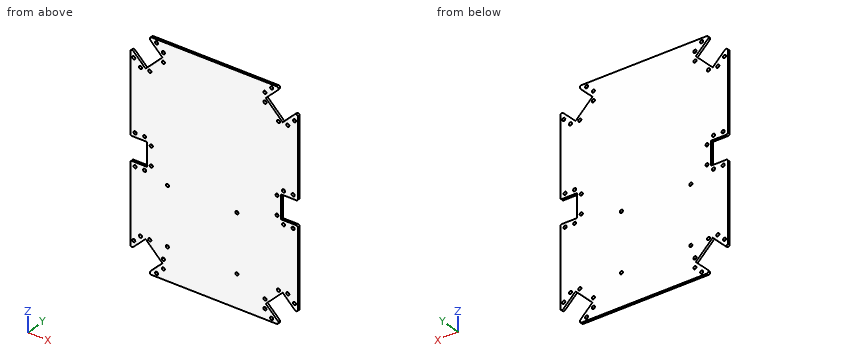
```python
from build123d import *

# Parameters (mm, degrees)
SKETCH2_W           = 140
SKETCH2_H           = 190
SKETCH2_R           = 1.3
BOSS_EXTRUDE1_DEPTH = 2
SKETCH3_W           = 14
SKETCH3_H           = 20
CUT_EXTRUDE1_DEPTH  = 2
FILLET1_R           = 1.5
SKETCH4_R           = 1.3
CUT_EXTRUDE2_DEPTH  = 2


with BuildPart() as part:
    # Sketch2 → Boss-Extrude1 (new body)
    with BuildSketch(Plane(origin=(0, 0, 0), x_dir=(1, 0, 0), z_dir=(0, 1, 0))):
        Rectangle(SKETCH2_W, SKETCH2_H)
        with Locations(Location((42.422835534, 78.736544033, 0), (0, 0, 270))):
            Circle(SKETCH2_R, mode=Mode.SUBTRACT)
        with Locations(Location((42.422835534, 86.514718626, 0), (0, 0, 270))):
            Circle(SKETCH2_R, mode=Mode.SUBTRACT)
        with Locations(Location((48.079689783, 92.171572875, 0), (0, 0, 270))):
            Circle(SKETCH2_R, mode=Mode.SUBTRACT)
        with Locations(Location((66, 13.5, 0), (0, 0, 270))):
            Circle(SKETCH2_R, mode=Mode.SUBTRACT)
        with Locations(Location((58, 13.5, 0), (0, 0, 270))):
            Circle(SKETCH2_R, mode=Mode.SUBTRACT)
        with Locations(Location((52.5, 8, 0), (0, 0, 270))):
            Circle(SKETCH2_R, mode=Mode.SUBTRACT)
        with Locations(Location((52.5, -8, 0), (0, 0, 90))):
            Circle(SKETCH2_R, mode=Mode.SUBTRACT)
        with Locations(Location((58, -13.5, 0), (0, 0, 90))):
            Circle(SKETCH2_R, mode=Mode.SUBTRACT)
        with Locations(Location((66, -13.5, 0), (0, 0, 90))):
            Circle(SKETCH2_R, mode=Mode.SUBTRACT)
        with Locations(Location((67.171572875, 73.079689783, 0), (0, 0, 90))):
            Circle(SKETCH2_R, mode=Mode.SUBTRACT)
        with Locations(Location((61.514718626, 67.422835534, 0), (0, 0, 90))):
            Circle(SKETCH2_R, mode=Mode.SUBTRACT)
        with Locations(Location((53.736544033, 67.422835534, 0), (0, 0, 90))):
            Circle(SKETCH2_R, mode=Mode.SUBTRACT)
        with Locations(Location((67.171572875, -73.079689783, 0), (0, 0, 270))):
            Circle(SKETCH2_R, mode=Mode.SUBTRACT)
        with Locations(Location((61.514718626, -67.422835534, 0), (0, 0, 270))):
            Circle(SKETCH2_R, mode=Mode.SUBTRACT)
        with Locations(Location((53.736544033, -67.422835534, 0), (0, 0, 270))):
            Circle(SKETCH2_R, mode=Mode.SUBTRACT)
        with Locations(Location((48.079689783, -92.171572875, 0), (0, 0, 90))):
            Circle(SKETCH2_R, mode=Mode.SUBTRACT)
        with Locations(Location((42.422835534, -86.514718626, 0), (0, 0, 90))):
            Circle(SKETCH2_R, mode=Mode.SUBTRACT)
        with Locations(Location((42.422835534, -78.736544033, 0), (0, 0, 90))):
            Circle(SKETCH2_R, mode=Mode.SUBTRACT)
        with Locations(Location((-48.079689783, 92.171572875, 0), (0, 0, 90))):
            Circle(SKETCH2_R, mode=Mode.SUBTRACT)
        with Locations(Location((-42.422835534, 86.514718626, 0), (0, 0, 90))):
            Circle(SKETCH2_R, mode=Mode.SUBTRACT)
        with Locations(Location((-42.422835534, 78.736544033, 0), (0, 0, 90))):
            Circle(SKETCH2_R, mode=Mode.SUBTRACT)
        with Locations(Location((-67.171572875, 73.079689783, 0), (0, 0, 270))):
            Circle(SKETCH2_R, mode=Mode.SUBTRACT)
        with Locations(Location((-61.514718626, 67.422835534, 0), (0, 0, 270))):
            Circle(SKETCH2_R, mode=Mode.SUBTRACT)
        with Locations(Location((-53.736544033, 67.422835534, 0), (0, 0, 270))):
            Circle(SKETCH2_R, mode=Mode.SUBTRACT)
        with Locations(Location((-67.171572875, -73.079689783, 0), (0, 0, 90))):
            Circle(SKETCH2_R, mode=Mode.SUBTRACT)
        with Locations(Location((-61.514718626, -67.422835534, 0), (0, 0, 90))):
            Circle(SKETCH2_R, mode=Mode.SUBTRACT)
        with Locations(Location((-53.736544033, -67.422835534, 0), (0, 0, 90))):
            Circle(SKETCH2_R, mode=Mode.SUBTRACT)
        with Locations(Location((-42.422835534, -78.736544033, 0), (0, 0, 270))):
            Circle(SKETCH2_R, mode=Mode.SUBTRACT)
        with Locations(Location((-42.422835534, -86.514718626, 0), (0, 0, 270))):
            Circle(SKETCH2_R, mode=Mode.SUBTRACT)
        with Locations(Location((-48.079689783, -92.171572875, 0), (0, 0, 270))):
            Circle(SKETCH2_R, mode=Mode.SUBTRACT)
        with Locations(Location((-52.5, -8, 0), (0, 0, 270))):
            Circle(SKETCH2_R, mode=Mode.SUBTRACT)
        with Locations(Location((-58, -13.5, 0), (0, 0, 270))):
            Circle(SKETCH2_R, mode=Mode.SUBTRACT)
        with Locations(Location((-66, -13.5, 0), (0, 0, 270))):
            Circle(SKETCH2_R, mode=Mode.SUBTRACT)
        with Locations(Location((-66, 13.5, 0), (0, 0, 90))):
            Circle(SKETCH2_R, mode=Mode.SUBTRACT)
        with Locations(Location((-58, 13.5, 0), (0, 0, 90))):
            Circle(SKETCH2_R, mode=Mode.SUBTRACT)
        with Locations(Location((-52.5, 8, 0), (0, 0, 90))):
            Circle(SKETCH2_R, mode=Mode.SUBTRACT)
    extrude(amount=BOSS_EXTRUDE1_DEPTH)

    # Sketch3 → Cut-Extrude1 (cut)
    with BuildSketch(Plane(origin=(0, 2, 0), x_dir=(1, 0, 0), z_dir=(0, 1, 0))):
        with Locations((63, 0)):
            Rectangle(SKETCH3_W, SKETCH3_H)
        Polygon((55.857864376, 95), (43.129942315, 82.272077939), (57.272077939, 68.129942315), (70, 80.857864376), (70, 95), align=None)
        Polygon((70, -80.857864376), (70, -95), (55.857864376, -95), (43.129942315, -82.272077939), (57.272077939, -68.129942315), align=None)
        Polygon((-70, 80.857864376), (-70, 95), (-55.857864376, 95), (-43.129942315, 82.272077939), (-57.272077939, 68.129942315), align=None)
        with Locations((-63, 0)):
            Rectangle(SKETCH3_W, SKETCH3_H)
        Polygon((-57.272077939, -68.129942315), (-70, -80.857864376), (-70, -95), (-55.857864376, -95), (-43.129942315, -82.272077939), align=None)
    extrude(amount=-CUT_EXTRUDE1_DEPTH, mode=Mode.SUBTRACT)

    # Fillet1
    fillet1_edges = [part.edges().sort_by_distance(p)[0] for p in [
        (55.857864376, 1, -95),
        (70, 1, -80.857864376),
        (70, 1, 80.857864376),
        (55.857864376, 1, 95),
        (-70, 1, -80.857864376),
        (-55.857864376, 1, -95),
        (-70, 1, 10),
        (-70, 1, -10),
        (-55.857864376, 1, 95),
        (-70, 1, 80.857864376),
        (70, 1, -10),
        (70, 1, 10),
    ]]
    fillet(fillet1_edges, radius=FILLET1_R)

    # Sketch4 → Cut-Extrude2 (cut)
    with BuildSketch(Plane(origin=(0, 2, 0), x_dir=(1, 0, 0), z_dir=(0, 1, 0))):
        with Locations(Location((-39, 67.5, 0), (0, 0, 270))):
            Circle(SKETCH4_R)
        with Locations(Location((19, 67.5, 0), (0, 0, 270))):
            Circle(SKETCH4_R)
        with Locations(Location((19, 18.5, 0), (0, 0, 270))):
            Circle(SKETCH4_R)
        with Locations(Location((-39, 18.5, 0), (0, 0, 270))):
            Circle(SKETCH4_R)
    extrude(amount=-CUT_EXTRUDE2_DEPTH, mode=Mode.SUBTRACT)


solid = part.part
```
Source: CAD feature listing. Evaluate the final solid. Frame: model axes, mm. Coordinates: 2 decimals unless noted, no trailing zeros. Loops run counter-clockwise (first coordinate to the right, second up) from the corner with the lowest first, then second, coordinate; pieces in that order, holes last. Notation, with made-up numbers: M 86.25,36 L 111.25,36 A26 ccw 111.25,66 Z; hole C 9,14 d9. An arc over 180 degrees is marked long. Use a Markdown table: item, result. Add a question column.
Q1. Section query B-B, the plane y = 0.3. State how many separate pieces and enclosed holes the cut face has, and give its area (3 significant figures).
Q2. Section query A-A, the plane z = -1.5. Return loops of the section in (x, y), and give its area (3 significant figures).
Q3. Material intervals for L1, parallel to X at y = 0.6, z = -76; L2, parallel to X at y = 1.5, z = 8; L3, parallel to Z at x = -54, y = 1.4, sorted ascending.
Q4. First-contact query: pin 1 (1.6 mm diameter, centred on x = -67.17, z = 73.08, fed in from +Y). Flat tip, straight axial feed; report the tip coordinate or a pass-through.
Result:
| question | item | result |
|---|---|---|
| 1 | separate pieces | 1 |
| 1 | enclosed holes | 40 |
| 1 | area | 24,000 mm2 |
| 2 | outline | M -56,0 L 56,0 L 56,2 L -56,2 Z |
| 2 | area | 224 mm2 |
| 3 | L1 | x = -70 to -65.14, -49.4 to 49.4, 65.14 to 70 |
| 3 | L2 | x = -56 to -53.8, -51.2 to 51.2, 53.8 to 56 |
| 3 | L3 | z = -71.4 to -68.7, -66.15 to 66.15, 68.7 to 71.4 |
| 4 | pin 1 | passes through |
